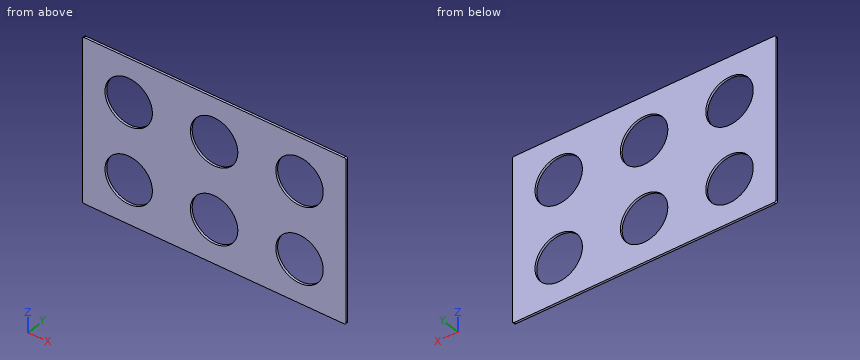
from build123d import *

# Parameters (mm, degrees)
SKETCH1_W           = 368.3
SKETCH1_H           = 228.6
SKETCH1_R           = 33.147
BOSS_EXTRUDE1_DEPTH = 3.175
FILLET1_R           = 2.54


with BuildPart() as part:
    # Sketch1 → Boss-Extrude1 (new body)
    with BuildSketch(Plane(origin=(0, 0, 0), x_dir=(1, 0, 0), z_dir=(0, 1, 0))):
        Rectangle(SKETCH1_W, SKETCH1_H)
        with Locations(Location((119.38, 53.5305, 0), (0, 0, 270))):
            Circle(SKETCH1_R, mode=Mode.SUBTRACT)
        with Locations(Location((0, 53.5305, 0), (0, 0, 270))):
            Circle(SKETCH1_R, mode=Mode.SUBTRACT)
        with Locations(Location((-119.38, 53.5305, 0), (0, 0, 270))):
            Circle(SKETCH1_R, mode=Mode.SUBTRACT)
        with Locations(Location((-119.38, -53.5305, 0), (0, 0, 270))):
            Circle(SKETCH1_R, mode=Mode.SUBTRACT)
        with Locations(Location((0, -53.5305, 0), (0, 0, 270))):
            Circle(SKETCH1_R, mode=Mode.SUBTRACT)
        with Locations(Location((119.38, -53.5305, 0), (0, 0, 270))):
            Circle(SKETCH1_R, mode=Mode.SUBTRACT)
    extrude(amount=BOSS_EXTRUDE1_DEPTH)

    # Fillet1
    fillet1_edges = [part.edges().sort_by_distance(p)[0] for p in [
        (184.15, 1.5875, 114.3),
        (-184.15, 1.5875, 114.3),
        (-184.15, 1.5875, -114.3),
        (184.15, 1.5875, -114.3),
    ]]
    fillet(fillet1_edges, radius=FILLET1_R)


solid = part.part
Geometry: final body of the model. Coordinates: model frame, mm. Round coordinates to 2 decimals unless told otherwise and drop trailing zeros. Order: outer loops, then holes, each group sorted by start corner. A loop starts at its lowest first (then second) coordinate and runs counter-clockwise, first axis right, second up. Notation, with made-up numbers: (39.5, 15) - (94.5, 15) arc R33 ccw to (94.5, 46) - close; hole circle Ø6 at (-24, 13.5). An arc over 180 degrees is marked (long way). Write each question's results on one line, items separated by ' | '.
Item 1: Section D-D, the plane z = 76. Return the cut outline in (x, y) (3 decimals).
Completed:
outline: (-184.15, 0) - (-143.749, 0) - (-143.749, 3.175) - (-184.15, 3.175) - close; (-95.011, 0) - (-24.369, 0) - (-24.369, 3.175) - (-95.011, 3.175) - close; (24.369, 0) - (95.011, 0) - (95.011, 3.175) - (24.369, 3.175) - close; (143.749, 0) - (184.15, 0) - (184.15, 3.175) - (143.749, 3.175) - close
Item 2: Material intervals for line 1 along X through (y, z) = (3, -54); line 2 along X through (y, z) = (0.85, 55.5); line 3 along Z through (x, y) = (131.5, 0.2), sorted ascending. Write a range as [from, to].
Completed:
line 1: [-184.15, -152.52], [-86.24, -33.14], [33.14, 86.24], [152.52, 184.15] | line 2: [-184.15, -152.47], [-86.29, -33.09], [33.09, 86.29], [152.47, 184.15] | line 3: [-114.3, -84.38], [-22.68, 22.68], [84.38, 114.3]
Item 3: Section C-C, the plane z = -59.5. Return the cut outline in (x, y) (3 decimals), and give its area (3 significant figures).
Completed:
outline: (-184.15, 0) - (-151.985, 0) - (-151.985, 3.175) - (-184.15, 3.175) - close; (-86.775, 0) - (-32.605, 0) - (-32.605, 3.175) - (-86.775, 3.175) - close; (32.605, 0) - (86.775, 0) - (86.775, 3.175) - (32.605, 3.175) - close; (151.985, 0) - (184.15, 0) - (184.15, 3.175) - (151.985, 3.175) - close | area: 548 mm^2
Item 4: Section B-B, the plane y = 2.15. Return the cut outline in (x, z), and give its area (3 significant figures).
Completed:
outline: (-184.15, -111.76) arc R2.54 ccw to (-181.61, -114.3) - (181.61, -114.3) arc R2.54 ccw to (184.15, -111.76) - (184.15, 111.76) arc R2.54 ccw to (181.61, 114.3) - (-181.61, 114.3) arc R2.54 ccw to (-184.15, 111.76) - close; hole circle Ø66.29 at (-119.38, -53.53); hole circle Ø66.29 at (-119.38, 53.53); hole circle Ø66.29 at (0, -53.53); hole circle Ø66.29 at (0, 53.53); hole circle Ø66.29 at (119.38, -53.53); hole circle Ø66.29 at (119.38, 53.53) | area: 63,500 mm^2
Item 5: Section A-A, the plane x = 119.38. Return the cut outline in (y, z) (1 decimal), and give its area (3 significant figures).
Completed:
outline: (0, -114.3) - (3.2, -114.3) - (3.2, -86.7) - (0, -86.7) - close; (0, -20.4) - (3.2, -20.4) - (3.2, 20.4) - (0, 20.4) - close; (0, 86.7) - (3.2, 86.7) - (3.2, 114.3) - (0, 114.3) - close | area: 305 mm^2
